Part print with two shaded views. Sizes in mm from the minimum x, y, z corner. A direction names the side the tool comes from. Coordinates: 2 decimals unless noted, no trailing zeros. Order: outer loops, then holes, each group sorted by start corner. A loop starts at its lowest first (then second) coordinate and runs counter-clockwise, first axis right, second up.
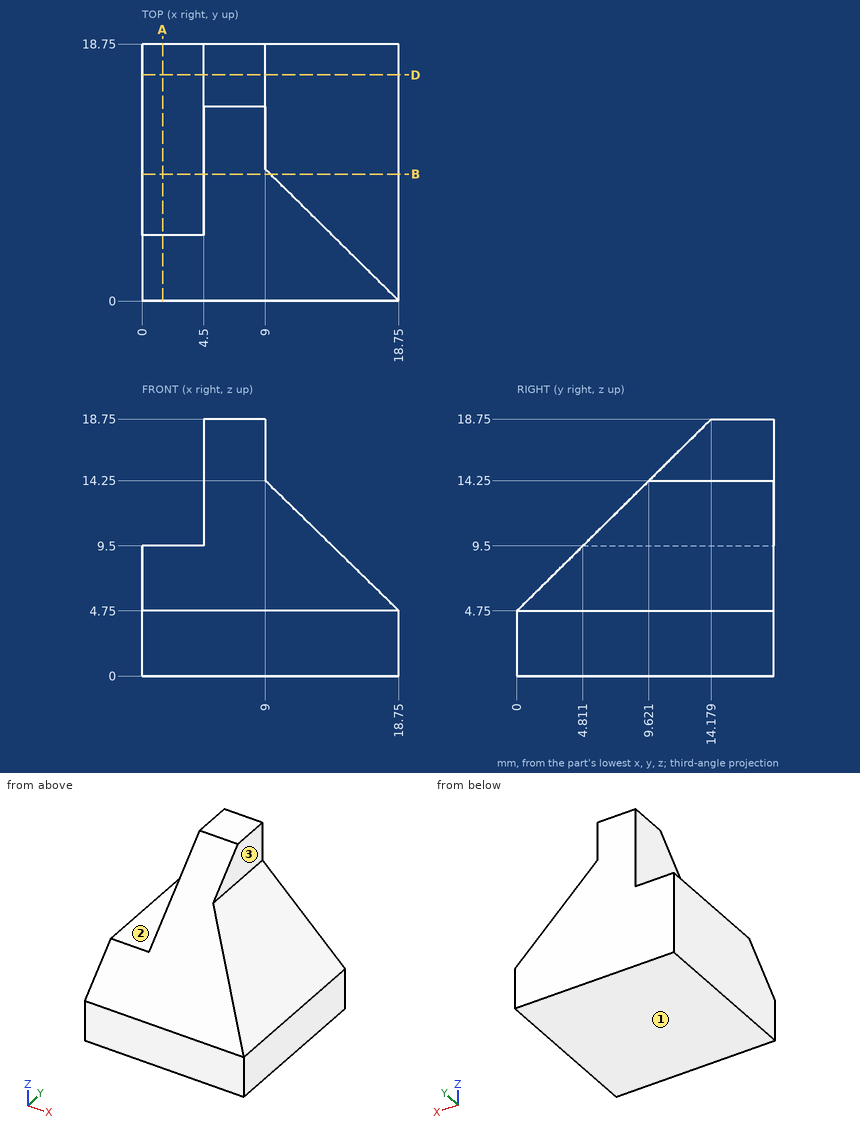
Q1. Pin check, flat tips, straight feed: pin 1 Ø5 at (x, y) = (7.5, 4) entering from +Z; pin 2 Ø5 at (x, y) = (2.5, 10.5) entering from +Z; pin 3 Ø10 at (x, y) = (4.5, 4.5) entering from -Z; pin 4 Ø3.5 at (y, z) = (15.5, 16.5) entering from +X. Stop position of each tip, or through.
Results list:
pin 1: stops at z = 11.17
pin 2: stops at z = 16.6
pin 3: stops at z = 0
pin 4: stops at x = 9
Q2. Cut at D-D on y = 16.5. Write the cut outline in (x, z).
Results list:
outline: (0, 0) - (18.75, 0) - (18.75, 4.75) - (9, 14.25) - (9, 18.75) - (4.5, 18.75) - (4.5, 9.5) - (0, 9.5) - close
Q3. Wall check: line 1 along X through (y, z) = (17.5, 15.5); line 2 along Z through (x, y) = (2.5, 11.75); line 3 along X through (y, z) = (7, 7.5). Give the ranges that are in metal, low to high.
Results list:
line 1: x = 4.5 to 9
line 2: z = 0 to 9.5
line 3: x = 0 to 15.93
Q4. Cut at B-B on y = 9.25. Write the cut outline in (x, z), and give its area (3 significant figures).
Results list:
outline: (0, 0) - (18.75, 0) - (18.75, 4.75) - (9.38, 13.88) - (4.5, 13.88) - (4.5, 9.5) - (0, 9.5) - close
area: 198 mm2
Q5. Which spindle directions (+Z, -Z, +X, -X, +Y, -Y) get a long thin tool onto all of the face, cutting with end or side? Do the marked faces 1, 2 and 3. Say none if no direction does.
Results list:
face 1: -Z, +X, -X, +Y, -Y
face 2: +Z, -X, +Y, -Y
face 3: +Z, +X, +Y, -Y
Q6. Cut at A-A on x = 1.5. Write the cut outline in (y, z), and give its area (3 significant figures).
Results list:
outline: (0, 0) - (18.75, 0) - (18.75, 9.5) - (4.81, 9.5) - (0, 4.75) - close
area: 167 mm2
